```python
from build123d import *

# Parameters (mm, degrees)
F0_R     = 1.25
F1_DEPTH = 1.355102
F2_R     = 0.4
F3_R     = 1
F4_DEPTH = 18.831681
F5_DEPTH = 3
F6_R     = 1
F9_R     = 0.5


with BuildPart() as f1:
    # F0 (on Top) → F1 (new body)
    with BuildSketch(Plane.XY):
        Polygon((0, 12.436029), (-10, 12.436029), (-10, -7.563971), (0, -7.563971), (0, -4.463971), (4, -4.463971), (4, -1.163971), (0, -1.163971), (0, 2.336029), (4, 2.336029), (4, 5.636029), (0, 5.636029), (0, 9.136029), (4, 9.136029), (4, 12.436029), align=None)
        with Locations((-5, -3.563971)):
            Circle(F0_R, mode=Mode.SUBTRACT)
        with Locations((-5, 8.436029)):
            Circle(F0_R, mode=Mode.SUBTRACT)
    extrude(amount=F1_DEPTH)

    # F2
    f2_edges = [f1.edges().sort_by_distance(p)[0] for p in [
        (4, -2.813971, 1.355102),
        (4, 3.986029, 1.355102),
        (4, 10.786029, 1.355102),
        (4, -2.813971, 0),
        (4, 3.986029, 0),
        (4, 10.786029, 0),
    ]]
    fillet(f2_edges, radius=F2_R)


with BuildPart() as f4:
    # F3 (on Front) → F4 (new body, symmetric)
    with BuildSketch(Plane.XZ):
        with Locations((2, 1.5)):
            Circle(F3_R)
    extrude(amount=F4_DEPTH, both=True)


with BuildPart() as f5:
    # F0 (on Top) → F5 (new body)
    with BuildSketch(Plane.XY):
        Polygon((0, 12.436029), (-10, 12.436029), (-10, -7.563971), (0, -7.563971), (0, -4.463971), (4, -4.463971), (4, -1.163971), (0, -1.163971), (0, 2.336029), (4, 2.336029), (4, 5.636029), (0, 5.636029), (0, 9.136029), (4, 9.136029), (4, 12.436029), align=None)
        with Locations((-5, -3.563971)):
            Circle(F0_R, mode=Mode.SUBTRACT)
        with Locations((-5, 8.436029)):
            Circle(F0_R, mode=Mode.SUBTRACT)
    extrude(amount=F5_DEPTH)

    # F6
    f6_edges = [f5.edges().sort_by_distance(p)[0] for p in [
        (4, -2.813971, 3),
        (4, 3.986029, 3),
        (4, 10.786029, 3),
        (4, 10.786029, 0),
        (4, 3.986029, 0),
        (4, -2.813971, 0),
    ]]
    fillet(f6_edges, radius=F6_R)

    # F7: cut F4
    add(f4.part, mode=Mode.SUBTRACT)

    # F9
    f9_edges = [f5.edges().sort_by_distance(p)[0] for p in [
        (-6.25, -3.563971, 3),
        (-6.25, 8.436029, 3),
        (-6.25, -3.563971, 0),
        (-6.25, 8.436029, 0),
    ]]
    fillet(f9_edges, radius=F9_R)


solid = f5.part
```
Design review of the part built by this model. Coordinates are the model's own, in mm. A direction names the side the tool comes from. Round coordinates to 2 decimals unless told otherwise and drop trailing zeros. Write each loop counter-clockwise with the first axis right and the second up, starting at its lowest first coordinate (ties: lowest second). Pieces come first, ordered by that corner, then holes. Notation, with made-up numbers: (10.25, -16) -> (57.25, -16) arc R31 ccw to (57.25, 23) -> close; hole circle Ø5 at (-2.75, -6). An arc over 180 degrees is marked (long way). Write item = value, one per line. Start each with the question number.
1) Take a section at A-A, the plane z = 1.5. State the section outline as (x, y) points.
2) Mouldability with a two-part tool opening along Y and no side actions: class faces 4 (the face through (3.715, -2.791, 2.699)), 5 (the face through (1.08, 9.136, 0.81)), 6 (the face through (0, 7, 1)), 7 (the face through (1.08, -4.464, 0.81)) as +Y half, -Y half, draft (parallel to the pull), parting line (faces both ways), or undercut.
3) Take a section at B-B, the plane x = 2. State the section outline as (y, z) points.
4) Take a section at C-C, the plane x = -5. State the section outline as (y, z) points, plus the area to 3 significant figures.
5) Clearance check with a flat-ended pin moving along its axis: pin 1 (1.5 mm diameter, centred on y = -6, z = 1, fed in from +X). State where the tip first meets the part, or that it passes through.
6) Tool access review of faces 1 (the face through (1.2, 10.8, 0.9)), 2 (the face through (0, -6, 1)), 3 (the face through (1.08, 2.336, 0.81)): name each direction out of +Z, -Z, +X, -X, +Y, -Y from which nothing blocks a thin tool from reaching the whole face with its end or side.
7) Wall thickness on probe 1 along Y at (x, z) = (0.25, 2.55); probe 2 along Z at (x, y) = (2, 11.4); probe 3 along Y at (x, z) = (-4.75, 0.25): over which ranges is each line inside the solid? List them lowest first. Write a range as from..to.
8) Take a section at D-D, the plane y = 11.25. State the section outline as (x, z) points.
Results list:
q1.outline = (-10, -7.56) -> (0, -7.56) -> (0, -4.46) -> (1, -4.46) -> (1, -1.16) -> (0, -1.16) -> (0, 2.34) -> (1, 2.34) -> (1, 5.64) -> (0, 5.64) -> (0, 9.14) -> (1, 9.14) -> (1, 12.44) -> (-10, 12.44) -> close; (3, -4.46) -> (4, -4.46) -> (4, -1.16) -> (3, -1.16) -> close; (3, 2.34) -> (4, 2.34) -> (4, 5.64) -> (3, 5.64) -> close; (3, 9.14) -> (4, 9.14) -> (4, 12.44) -> (3, 12.44) -> close; hole circle Ø2.5 at (-5, -3.56); hole circle Ø2.5 at (-5, 8.44)
q2.face_4 = draft
q2.face_5 = undercut
q2.face_6 = undercut
q2.face_7 = -Y half
q3.outline = (-4.46, 0) -> (-1.16, 0) -> (-1.16, 0.5) -> (-4.46, 0.5) -> close; (-4.46, 2.5) -> (-1.16, 2.5) -> (-1.16, 3) -> (-4.46, 3) -> close; (2.34, 0) -> (5.64, 0) -> (5.64, 0.5) -> (2.34, 0.5) -> close; (2.34, 2.5) -> (5.64, 2.5) -> (5.64, 3) -> (2.34, 3) -> close; (9.14, 0) -> (12.44, 0) -> (12.44, 0.5) -> (9.14, 0.5) -> close; (9.14, 2.5) -> (12.44, 2.5) -> (12.44, 3) -> (9.14, 3) -> close
q4.outline = (-7.56, 0) -> (-5.31, 0) arc R0.5 ccw to (-4.81, 0.5) -> (-4.81, 2.5) arc R0.5 ccw to (-5.31, 3) -> (-7.56, 3) -> close; (-2.31, 0.5) arc R0.5 ccw to (-1.81, 0) -> (6.69, 0) arc R0.5 ccw to (7.19, 0.5) -> (7.19, 2.5) arc R0.5 ccw to (6.69, 3) -> (-1.81, 3) arc R0.5 ccw to (-2.31, 2.5) -> close; (9.69, 0.5) arc R0.5 ccw to (10.19, 0) -> (12.44, 0) -> (12.44, 3) -> (10.19, 3) arc R0.5 ccw to (9.69, 2.5) -> close
q4.area = 44.6 mm²
q5.pin_1 = 0
q6.face_1 = +Y, -Y
q6.face_2 = +Z, -Z, +X, -Y
q6.face_3 = +Z, -Z, +X
q7.probe_1 = -4.46..-1.16, 2.34..5.64, 9.14..12.44
q7.probe_2 = 0..0.5, 2.5..3
q7.probe_3 = -7.56..-4.86, -2.27..7.14, 9.73..12.44
q8.outline = (-10, 0) -> (3, 0) arc R1 ccw to (4, 1) -> (4, 2) arc R1 ccw to (3, 3) -> (-10, 3) -> close; hole circle Ø2 at (2, 1.5)
